```python
from build123d import *

# Parameters (mm, degrees)
F0_W      = 42.3
F0_H      = 42.3
F1_DEPTH  = 40
F2_R      = 11
F3_DEPTH  = 2
F4_R      = 4
F5_DEPTH  = 300
F6_SIZE   = 4
F9_DEPTH  = 7.5
F10_R     = 1.5
F11_DEPTH = 10


with BuildPart() as f1:
    # F0 (on Front) → F1 (new body)
    with BuildSketch(Plane.XZ):
        Rectangle(F0_W, F0_H)
    extrude(amount=F1_DEPTH)

    # F2 (on face) → F3 (join)
    with BuildSketch(Plane(origin=(0, 0, 0), x_dir=(-1, 0, 0), z_dir=(0, 1, 0))):
        Circle(F2_R)
    extrude(amount=F3_DEPTH)

    # F4 (on face) → F5 (join)
    with BuildSketch(Plane(origin=(0, 2, 0), x_dir=(-1, 0, 0), z_dir=(0, 1, 0))):
        Circle(F4_R)
    extrude(amount=F5_DEPTH)

    # F6
    f6_edges = [f1.edges().sort_by_distance(p)[0] for p in [
        (-21.15, -20, 21.15),
        (-21.15, -20, -21.15),
        (21.15, -20, -21.15),
        (21.15, -20, 21.15),
    ]]
    chamfer(f6_edges, length=F6_SIZE)

    # F8 (on offset) → F9 (cut, symmetric)
    with BuildSketch(Plane.XZ.offset(20)):
        with BuildLine():
            ThreePointArc((14.3215728753, 21.15), (19.15, 19.15), (21.15, 14.3215728753))
            Line((21.15, 14.3215728753), (21.15, 21.15))
            Line((21.15, 21.15), (14.3215728753, 21.15))
        make_face()
        with BuildLine():
            Line((-21.15, 21.15), (-21.15, 14.3215728753))
            ThreePointArc((-21.15, 14.3215728753), (-19.15, 19.15), (-14.3215728753, 21.15))
            Line((-14.3215728753, 21.15), (-21.15, 21.15))
        make_face()
        with BuildLine():
            Line((21.15, -21.15), (21.15, -14.3215728753))
            ThreePointArc((21.15, -14.3215728753), (19.15, -19.15), (14.3215728753, -21.15))
            Line((14.3215728753, -21.15), (21.15, -21.15))
        make_face()
        with BuildLine():
            ThreePointArc((-14.3215728753, -21.15), (-19.15, -19.15), (-21.15, -14.3215728753))
            Line((-21.15, -14.3215728753), (-21.15, -21.15))
            Line((-21.15, -21.15), (-14.3215728753, -21.15))
        make_face()
    extrude(amount=F9_DEPTH, both=True, mode=Mode.SUBTRACT)

    # F10 (on face) → F11 (cut)
    with BuildSketch(Plane(origin=(0, 0, 0), x_dir=(-1, 0, 0), z_dir=(0, 1, 0))):
        with Locations((-15.5, 15.5)):
            Circle(F10_R)
        with Locations((15.5, 15.5)):
            Circle(F10_R)
        with Locations((-15.5, -15.5)):
            Circle(F10_R)
        with Locations((15.5, -15.5)):
            Circle(F10_R)
    extrude(amount=-F11_DEPTH, mode=Mode.SUBTRACT)


solid = f1.part
```
Geometry check sheet. Reference: the model listing, model coordinates, mm. A direction names the side the tool comes from. Coordinates: 2 decimals unless noted, no trailing zeros. Loops run counter-clockwise (first coordinate to the right, second up) from the corner with the lowest first, then second, coordinate; pieces in that order, holes last.
Item 1: Sectioned sample at A-A, the plane z = 0. Record the boundary of the cut face in (x, y), then the cut area to 3 significant figures.
Item 2: Release check for a two-part mould opening along Y. For faces 5 (the face through (-21.15, -20, 0)), 6 (the face through (0, 302, 0)), 7 (the face through (19.1, -19.9, 19.2)) record: released by +Y, released by -Y, zero draft, split by the parting line, or undercut.
Item 3: Go/stop test with flat-tipped pins: pin 1 Ø1 at (x, z) = (20.5, -16.5) entering from +Y; pin 2 Ø2 at (x, y) = (-3.5, 102.5) entering from -Z; pin 3 Ø12 at (x, y) = (15.5, 32) entering from +Z; pin 4 Ø12 at (x, z) = (-14.5, -2) entering from +Y. Record where each tip stops, or that it passes through.
Item 4: Thickness scan on line 1 (Z direction, x = 15.5, y = -2.5); line 2 (Z direction, x = 15, y = -6); line 3 (Y direction, x = -0.5, z = -4.5). Record the ranges inside material, lowest first.
Item 5: Access from +Z, -Z, +X, -X, +Y, -Y to the whole of each face (thin tool, end or side, straight path). Record for faces 1 (the face through (-19.1, -20.1, -19.2)), 2 (the face through (2.38, 0.99, -10.74)), 3 (the face through (19.2, -19.9, -19.1)), 4 (the face through (-19.2, -19.9, 19.1)).
Item 6: Sectioned sample at B-B, the plane x = 0. Record the boundary of the cut face in (y, z).
Item 7: Sectioned sample at C-C, the plane y = 229. Record the boundary of the cut face in (x, z), then the cut area to 3 significant figures.
Check result:
1. outline: (-21.15, -40) - (21.15, -40) - (21.15, 0) - (11, 0) - (11, 2) - (4, 2) - (4, 302) - (-4, 302) - (-4, 2) - (-11, 2) - (-11, 0) - (-21.15, 0) - close
1. area: 4,140 mm2
2. face 5: zero draft
2. face 6: released by +Y
2. face 7: undercut
3. pin 1: stops at y = 0
3. pin 2: stops at z = -3.12
3. pin 3: passes through
3. pin 4: stops at y = 2
4. line 1: z = -21.15 to -17, -14 to 14, 17 to 21.15
4. line 2: z = -21.15 to -16.91, -14.09 to 14.09, 16.91 to 21.15
4. line 3: y = -40 to 2
5. face 1: -Z, -X
5. face 2: +Y
5. face 3: -Z, +X
5. face 4: +Z, -X
6. outline: (-40, -21.15) - (0, -21.15) - (0, -11) - (2, -11) - (2, -4) - (302, -4) - (302, 4) - (2, 4) - (2, 11) - (0, 11) - (0, 21.15) - (-40, 21.15) - close
7. outline: circle Ø8 at (0, 0)
7. area: 50.3 mm2
